Geometry: final body of the model. Coordinates: model frame, mm. A direction names the side the tool comes from. Give positions to 0.01 mm unless a question says otherwise; leave off trailing zeros. Write each loop counter-clockwise with the first axis right and the second up, starting at its lowest first coordinate (ties: lowest second). Pieces come first, ordered by that corner, then holes. Notation, with made-up numbers: (-11, -21) -> (-6, -21) arc R29 ccw to (-6, 8) -> close; hole circle Ø6 at (49, 21). An arc over 180 degrees is marked (long way). Answer in a Markdown table with one row per item. Add a question column.
Item 1: Draft query along X for faces 4 (the flat face through (-12.775, -11, -1)), 5 (the cylindrical face through (-35.918, 18.17, -0.986)), 6 (the flat face through (-23, 20, -2)). Return one class per face: +X half, -X half, draft (parallel to the pull), parting line (faces both ways), or undercut.
Item 2: First-contact query: P1, Ø1, axis at y = 20, z = -1, coming from the -X side; P2, Ø12, axis at x = -36.5, y = -6.5, coming from the -Z side; P3, Ø1, axis at y = -12, z = -1, coming from the +X side (3 decimals); P4, Ø1, axis at y = 48.5, z = -1.5, coming from the -X side. Flat tips, straight axial feed; report the tip coordinate or a pass-through.
Item 3: Access query for faces 1 (the cylindrical face through (-25.07, 18.32, -0.99)), 2 (the flat face through (-20.501, 48, -1)), 3 (the flat face through (-12.775, 49, -1)). Directions: +Z, -Z, +X, -X, +Y, -Y. A direction counts if a zero-diameter tool reaches every point of the face in a straight line with its end or side. Return the directions, or none.
Item 4: Section query B-B on z = -0.95. Output: boundary loops of the cut face in (x, y), plus the area to 3 significant figures.
Item 5: Material intervals for probe 1 along X at (y, z) = (1, -0.1); probe 2 along X at (y, z) = (22, -0.3); probe 3 along Y at (x, z) = (-31, -1.65), sorted ascending. Write a range as from..to.
Item 6: Section query A-A on x = -26. Output: boundary loops of the cut face in (y, z).
Item 7: Section query C-C on y = 36.5. Output: boundary loops of the cut face in (x, z).
Item 8: Section query D-D on y = 25.5. Output: boundary loops of the cut face in (x, z).
```python
from build123d import *

# Parameters (mm, degrees)
F1_DEPTH = 2
F3_DEPTH = 4


with BuildPart() as f1:
    # F0 (on Top) → F1 (new body)
    with BuildSketch(Plane.XY):
        with BuildLine():
            Line((-11.113913, -8.946678), (-11.113913, 45.908373))
            ThreePointArc((-11.113913, 45.908373), (-11.943595, 45.97737), (-12.774983, 46.021273))
            Line((-12.774983, 46.021273), (-12.774983, 51.942695))
            ThreePointArc((-12.774983, 51.942695), (-16.661516, 51.777692), (-20.500943, 51.152251))
            Line((-20.500943, 51.152251), (-20.500943, 45.216891))
            ThreePointArc((-20.500943, 45.216891), (-41.372447, 18.480848), (-20.500943, -8.255196))
            Line((-20.500943, -8.255196), (-20.500943, -12.646276))
            ThreePointArc((-20.500943, -12.646276), (-16.661516, -13.271717), (-12.774983, -13.436719))
            Line((-12.774983, -13.436719), (-12.774983, -9.059578))
            ThreePointArc((-12.774983, -9.059578), (-11.943595, -9.015674), (-11.113913, -8.946678))
        make_face()
    extrude(amount=-F1_DEPTH)

    # F2 (on Top) → F3 (cut)
    with BuildSketch(Plane.XY):
        with BuildLine():
            Line((-14.205587, 10.137872), (-14.205587, 26.689431))
            ThreePointArc((-14.205587, 26.689431), (-22.497851, 18.413651), (-14.205587, 10.137872))
        make_face()
        with BuildLine():
            Line((-14.205587, 29.735729), (-14.205587, 32.172769))
            ThreePointArc((-14.205587, 32.172769), (-27.81698, 18.413651), (-14.205587, 4.654533))
            Line((-14.205587, 4.654533), (-14.205587, 7.396203))
            ThreePointArc((-14.205587, 7.396203), (-25.070721, 18.565966), (-14.205587, 29.735729))
        make_face()
        with BuildLine():
            ThreePointArc((-14.205587, 1.912864), (-30.605126, 18.515195), (-14.205587, 35.117526))
            Line((-14.205587, 35.117526), (-14.205587, 37.859194))
            ThreePointArc((-14.205587, 37.859194), (-33.448043, 18.616738), (-14.205587, -0.625718))
            Line((-14.205587, -0.625718), (-14.205587, 1.912864))
        make_face()
        with BuildLine():
            ThreePointArc((-14.205587, -3.196367), (-35.923159, 18.64843), (-14.205587, 40.493228))
            Line((-14.205587, 40.493228), (-14.205587, 43.230407))
            ThreePointArc((-14.205587, 43.230407), (-38.364807, 18.595791), (-14.205587, -6.038824))
            Line((-14.205587, -6.038824), (-14.205587, -3.196367))
        make_face()
    extrude(amount=-F3_DEPTH, mode=Mode.SUBTRACT)


solid = f1.part
```
Findings below:
| question | item | result |
|---|---|---|
| 1 | face 4 | +X half |
| 1 | face 5 | undercut |
| 1 | face 6 | draft |
| 2 | P1 | stops at x = -41.35 |
| 2 | P2 | passes through |
| 2 | P3 | stops at x = -12.775 |
| 2 | P4 | stops at x = -20.5 |
| 3 | face 1 | +Z, -Z |
| 3 | face 2 | +Z, -Z, -X, +Y |
| 3 | face 3 | +Z, -Z, +X, +Y |
| 4 | outline | (-20.5, -12.65) arc R32.69 ccw to (-12.77, -13.44) -> (-12.77, -9.06) arc R27.56 ccw to (-11.11, -8.95) -> (-11.11, 45.91) arc R27.56 ccw to (-12.77, 46.02) -> (-12.77, 51.94) arc R32.69 ccw to (-20.5, 51.15) -> (-20.5, 45.22) arc R27.56 ccw to (-20.5, -8.26) -> close; hole (-14.21, -6.04) -> (-14.21, -3.2) arc R21.85 cw to (-14.21, 40.49) -> (-14.21, 43.23) arc R24.64 ccw to start; hole (-14.21, -0.63) -> (-14.21, 1.91) arc R16.6 cw to (-14.21, 35.12) -> (-14.21, 37.86) arc R19.24 ccw to start; hole (-14.21, 4.65) -> (-14.21, 7.4) arc R11.17 cw to (-14.21, 29.74) -> (-14.21, 32.17) arc R13.76 ccw to start; hole (-14.21, 10.14) -> (-14.21, 26.69) arc R8.28 ccw to start |
| 4 | area | 868 mm^2 |
| 5 | probe 1 | x = -35.12..-30.97, -26.95..-21.95, -14.21..-11.11 |
| 5 | probe 2 | x = -41.15..-38.13, -35.66..-33.15, -30.24..-27.34, -24.53..-21.68, -14.21..-11.11 |
| 5 | probe 3 | y = -3.06..1.03, 4.83..9.22, 28.01..32.46, 36.17..40.02 |
| 6 | outline | (-6.24, -2) -> (-2.77, -2) -> (-2.77, 0) -> (-6.24, 0) -> close; (0.34, -2) -> (3.41, -2) -> (3.41, 0) -> (0.34, 0) -> close; (7.04, -2) -> (11.58, -2) -> (11.58, 0) -> (7.04, 0) -> close; (25.25, -2) -> (29.99, -2) -> (29.99, 0) -> (25.25, 0) -> close; (33.82, -2) -> (36.95, -2) -> (36.95, 0) -> (33.82, 0) -> close; (39.96, -2) -> (43.2, -2) -> (43.2, 0) -> (39.96, 0) -> close |
| 7 | outline | (-34.67, -2) -> (-30.65, -2) -> (-30.65, 0) -> (-34.67, 0) -> close; (-26.67, -2) -> (-21.31, -2) -> (-21.31, 0) -> (-26.67, 0) -> close; (-14.21, -2) -> (-11.11, -2) -> (-11.11, 0) -> (-14.21, 0) -> close |
| 8 | outline | (-40.46, -2) -> (-37.38, -2) -> (-37.38, 0) -> (-40.46, 0) -> close; (-34.82, -2) -> (-32.17, -2) -> (-32.17, 0) -> (-34.82, 0) -> close; (-29.06, -2) -> (-25.85, -2) -> (-25.85, 0) -> (-29.06, 0) -> close; (-22.66, -2) -> (-18.5, -2) -> (-18.5, 0) -> (-22.66, 0) -> close; (-14.21, -2) -> (-11.11, -2) -> (-11.11, 0) -> (-14.21, 0) -> close |
